from build123d import *

# Parameters (mm, degrees)
CHANFREIN1_SIZE = 0.5


with BuildPart() as part:
    # Esquisse1 → Base-Révolution (revolve)
    with BuildSketch(Plane.XY, mode=Mode.PRIVATE) as base_r_volution_sk:
        Polygon((0, 7.5), (5, 7.5), (5, 5.88), (29, 5.88), (29, 7.5), (34, 7.5), (34, 12.75), (10, 12.75), (10, 9.25), (8, 9.25), (8, 10), (0, 10), align=None)
    revolve(base_r_volution_sk.sketch.rotate(Axis((0, 0, 0), (1, 0, 0)), 90), axis=Axis((0, 0, 0), (1, 0, 0)))

    # Chanfrein1
    chanfrein1_edges = [part.edges().sort_by_distance(p)[0] for p in [
        (10, 0, -12.75),
        (0, 0, -10),
        (0, 0, -7.5),
        (34, 0, -7.5),
        (34, 0, -12.75),
    ]]
    chamfer(chanfrein1_edges, length=CHANFREIN1_SIZE)


solid = part.part
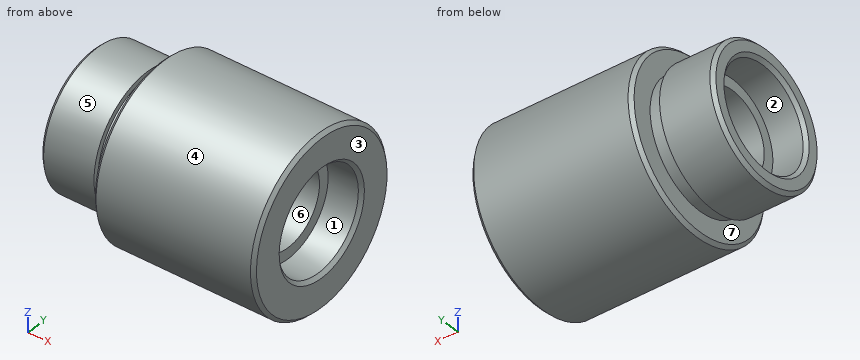
Part model, mm, in its own coordinate system. Face numbers are marked on the shaded views. A direction names the side the tool comes from. Coordinates: 2 decimals unless noted, no trailing zeros. Write each loop counter-clockwise with the first axis right and the second up, starting at its lowest first coordinate (ties: lowest second). Pieces come first, ordered by that corner, then holes. Notation, with made-up numbers: M -23,-22.5 L 21,-22.5 A30 ccw 21,7.5 Z; hole C 37.5,33 d7. An arc over 180 degrees is marked long. Return JSON: item names as keys, results as strings.
1. Probe L1, parallel to Y at x = 19, z = 0; L2, parallel to Y at x = 1.4, z = 0; L3, parallel to X at y = 1, z = 6.5. List the from-to ranges inside material, lowest first.
Determined:
{"L1": "-12.75 to -5.88, 5.88 to 12.75", "L2": "-10 to -7.5, 7.5 to 10", "L3": "5 to 29"}
2. 3-axis set-ups, long thin cutter, end or side, ignore diameter. For the marked faces 5, 6 and 7: which of +Z, -Z, +X, -X, +Y, -Y reach the whole face in a straight line?
Determined:
{"face 5": "-X", "face 6": "+X, -X", "face 7": "none"}
3. Pull direction Z, two halves, no side cores. Call the marked faces 1, 2, 3 and 4: pulls with the +Z half, pulls with the -Z half, needs draft (parallel to the pull), parting line crosses it, or undercut.
Determined:
{"face 1": "undercut", "face 2": "undercut", "face 3": "needs draft", "face 4": "parting line crosses it"}
4. Saw through at C-C, the plane x = 23.5. Write the cut outline in (y, z), then the cut area to 3 significant figures.
Determined:
{"outline": "C 0,0 d25.5; hole C 0,0 d11.76", "area": "402 mm²"}
5. Flat gauge pins, fed straight in: pin 1 Ø13.5 at (y, z) = (0, 0) entering from +X; pin 2 Ø2 at (y, z) = (2.5, 8.5) entering from -X; pin 3 Ø13.5 at (y, z) = (0, 0) entering from -X; pin 4 Ø6 at (x, y) = (10.5, 5.5) entering from -Z. Where does each tip first touch, or does it go through?
Determined:
{"pin 1": "x = 29", "pin 2": "x = 0", "pin 3": "x = 5", "pin 4": "z = -12.5"}
